from build123d import *

# Parameters (mm, degrees)
F1_DEPTH = 7
F2_R     = 3


# Not quite as in the source:
# - a feature names something its author has since deleted; it is built from what else it names


with BuildPart() as f1:
    # F0 (on Top) → F1 (new body)
    with BuildSketch(Plane.XY):
        with BuildLine():
            ThreePointArc((19.8306639352, -9.9816080654), (30.8415453201, -9.6036911235), (36.2407533076, 0))
            ThreePointArc((36.2407533076, 0), (30.8415453201, 9.6036911235), (19.8306639352, 9.9816080654))
            ThreePointArc((19.8306639352, 9.9816080654), (19.3470475071, 9.6503015364), (18.8215508103, 9.3904898984))
            ThreePointArc((18.8215508103, 9.3904898984), (13.7592466924, 0), (18.8215508103, -9.3904898984))
            ThreePointArc((18.8215508103, -9.3904898984), (19.3470475071, -9.6503015364), (19.8306639352, -9.9816080654))
        make_face()
        Polygon((31.3263880982, 3.8197050887), (31.4711556909, -3.5689602629), (25.1447675927, -7.3886653516), (18.6736119018, -3.8197050887), (18.5288443091, 3.5689602629), (24.8552324073, 7.3886653516), align=None, mode=Mode.SUBTRACT)
        with BuildLine():
            ThreePointArc((18.8215508103, -9.3904898984), (19.3184145947, -9.6991815224), (19.8306639352, -9.9816080654))
            ThreePointArc((19.8306639352, -9.9816080654), (19.3470475071, -9.6503015364), (18.8215508103, -9.3904898984))
        make_face()
        with BuildLine():
            ThreePointArc((18.8215508103, 9.3904898984), (19.3470475071, 9.6503015364), (19.8306639352, 9.9816080654))
            ThreePointArc((19.8306639352, 9.9816080654), (19.3184145947, 9.6991815224), (18.8215508103, 9.3904898984))
        make_face()
    extrude(amount=F1_DEPTH)

    # F2
    f2_edges = [f1.edges().sort_by_distance(p)[0] for p in [
        (31.178449, -9.39049, 7),
        (31.178449, -9.39049, 0),
    ]]
    fillet(f2_edges, radius=F2_R)


solid = f1.part
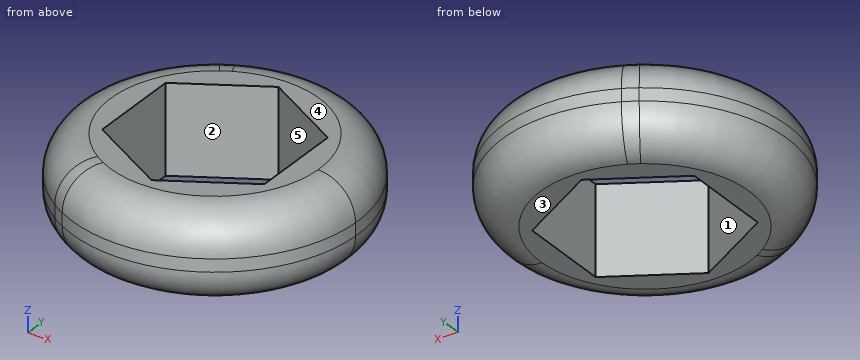
Build history of the part. All positions in model axes, mm. Face numbers are marked on the shaded views. A direction names the side the tool comes from. Coordinates: 2 decimals unless noted, no trailing zeros. Write each loop counter-clockwise with the first axis right and the second up, starting at its lowest first coordinate (ties: lowest second). Pieces come first, ordered by that corner, then holes.
(1) Drill centre lines: line 1 (Z direction, x = 33, y = -2.5); line 2 (Y direction, x = 26.5, z = 2.25); line 3 (X direction, y = -5.75, z = 5.5). Where is each one in solid material? Low to high.
(2) Cut at A-A on z = 0.75. List the corners of the cut face in (x, y), and give its area (3 significant figures).
(3) 3-axis set-ups, long thin cutter, end or side, ignore diameter. For the marked faces 4 and 5: which of +Z, -Z, +X, -X, +Y, -Y reach the whole face in a straight line?
(4) Cut at B-B on z = 5.75. List the corners of the cut face in (x, y).
(5) Pin check, flat tips, straight feed: pin 1 Ø1.5 at (x, z) = (24.5, 1) entering from -Y; pin 2 Ø1 at (x, z) = (29.5, 4) entering from +Y (3 decimals). Stop position of each tip, or through.
(6) Mould opens along X. For the marked faces 1, 2 and 3 say: pulls with the +X half, pulls with the -X half, needs draft (parallel to the pull), parting line crosses it, or undercut.
Working result:
1. line 1: z = 0 to 7
1. line 2: y = -11.04 to -6.57, 6.48 to 11.04
1. line 3: x = 15.81 to 22.17, 27.86 to 34.19
2. outline: circle Ø20.45 at (25, 0); hole (18.53, 3.57) - (18.67, -3.82) - (25.14, -7.39) - (31.47, -3.57) - (31.33, 3.82) - (24.86, 7.39) - close
2. area: 187 mm2
3. face 4: +Z, +X, -X, +Y, -Y
3. face 5: +Z, -Z
4. outline: circle Ø21.35 at (25, 0); hole (18.53, 3.57) - (18.67, -3.82) - (25.14, -7.39) - (31.47, -3.57) - (31.33, 3.82) - (24.86, 7.39) - close
5. pin 1: stops at y = -10.96
5. pin 2: stops at y = 10.505
6. face 1: undercut
6. face 2: undercut
6. face 3: needs draft
